```python
from build123d import *

# Parameters (mm, degrees)
F0_W     = 55.5
F0_H     = 27
F1_DEPTH = 15
F2_T     = -1.5
F3_R     = 2.5
F4_R     = 2.5


with BuildPart() as f1:
    # F0 (on Top) → F1 (new body)
    with BuildSketch(Plane.XY):
        Rectangle(F0_W, F0_H)
    extrude(amount=F1_DEPTH)

    # F2
    f2_openings = [f1.faces().sort_by_distance(p)[0] for p in [
        (0, 0, 15),
    ]]
    offset(amount=F2_T, openings=f2_openings)

    # F3
    f3_edges = [f1.edges().sort_by_distance(p)[0] for p in [
        (27.75, 13.5, 7.5),
        (-27.75, 13.5, 7.5),
        (27.75, -13.5, 7.5),
        (-27.75, -13.5, 7.5),
    ]]
    fillet(f3_edges, radius=F3_R)

    # F4
    f4_edges = [f1.edges().sort_by_distance(p)[0] for p in [
        (27.75, 0, 0),
        (27.017767, -12.767767, 0),
        (27.017767, 12.767767, 0),
        (0, -13.5, 0),
        (0, 13.5, 0),
        (-27.017767, -12.767767, 0),
        (-27.017767, 12.767767, 0),
        (-27.75, 0, 0),
    ]]
    fillet(f4_edges, radius=F4_R)


solid = f1.part
```
Source: CAD feature listing. Evaluate the final solid. Frame: model axes, mm. A direction names the side the tool comes from. Round coordinates to 2 decimals unless told otherwise and drop trailing zeros. Loops run counter-clockwise (first coordinate to the right, second up) from the corner with the lowest first, then second, coordinate; pieces in that order, holes last. Notation, with made-up numbers: M 53,-40 L 112,-40 A13 cw 112,-25 Z; hole C 77,-33 d1. An arc over 180 degrees is marked long. Put each result on its own line as item: value.
(1) Section A-A, the plane y = -4.5. Return loops of the section in (x, z), and give its area (3 significant figures).
Solutions:
outline: M -27.75,2.5 A2.5 ccw -25.25,0 L 25.25,0 A2.5 ccw 27.75,2.5 L 27.75,15 L 26.25,15 L 26.25,1.5 L -26.25,1.5 L -26.25,15 L -27.75,15 Z
area: 121 mm²
(2) Ray query, line 1 (Y direction, x = 7, z = 4); line 2 (X direction, y = -11.25, z = 12); line 3 (X direction, y = -10, z = 5). Return the intervals inside material, ascending. Write a range as [from, to].
Solutions:
line 1: [-13.5, -12], [12, 13.5]
line 2: [-27.74, -26.25], [26.25, 27.74]
line 3: [-27.75, -26.25], [26.25, 27.75]
(3) Section C-C, the plane x = 18.5. Return loops of the section in (y, z), and give its area (3 significant figures).
Solutions:
outline: M -13.5,2.5 A2.5 ccw -11,0 L 11,0 A2.5 ccw 13.5,2.5 L 13.5,15 L 12,15 L 12,1.5 L -12,1.5 L -12,15 L -13.5,15 Z
area: 78.3 mm²
(4) Section B-B, the plane z = 4.5. Return loops of the section in (x, y), and give its area (3 significant figures).
Solutions:
outline: M -27.75,-11 A2.5 ccw -25.25,-13.5 L 25.25,-13.5 A2.5 ccw 27.75,-11 L 27.75,11 A2.5 ccw 25.25,13.5 L -25.25,13.5 A2.5 ccw -27.75,11 Z; hole M -26.25,-12 L 26.25,-12 L 26.25,12 L -26.25,12 Z
area: 233 mm²
(5) Access query for faces 1 (the face through (27.75, 0, 9)), 2 (the face through (-26.25, 0, 8)). Directions: +Z, -Z, +X, -X, +Y, -Y. A direction counts if a zero-diameter tool reaches every point of the face in a straight line with its end or side. Return the directions, or none.
Solutions:
face 1: +Z, -Z, +X, +Y, -Y
face 2: +Z
